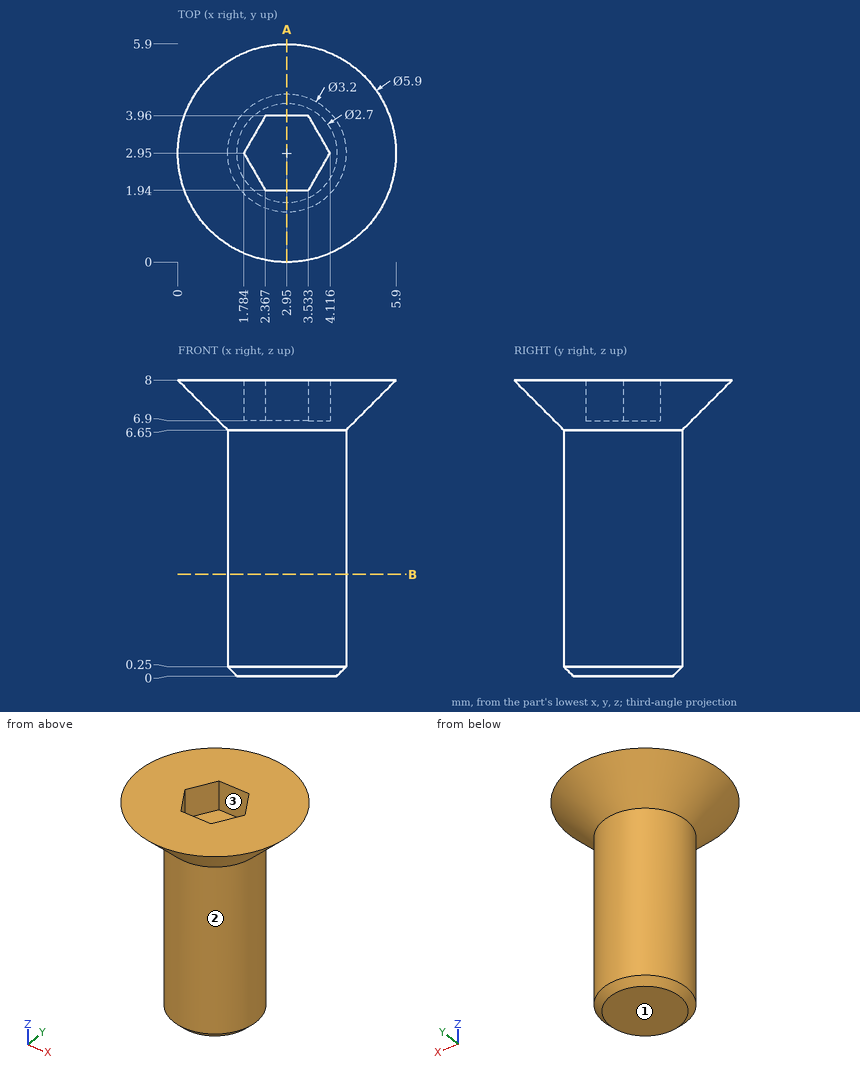
Design review of the part shown in the three views and the two pictorial views. Dimensions are in mm from the part's minimum x, y and z. A direction names the side the tool comes from. Coordinates: 2 decimals unless noted, no trailing zeros. Loops run counter-clockwise (first coordinate to the right, second up) from the corner with the lowest first, then second, coordinate; pieces in that order, holes last. Notation, with made-up numbers: (84.25, 21) - (89.25, 21) arc R25 ccw to (89.25, 46) - close; hole circle Ø6 at (65.25, 14.5). An arc over 180 degrees is marked (long way). Use a Markdown table: item, result. Add a question column.
Item 1: Tool access review of the marked faces 1, 2 and 3: name each direction out of +Z, -Z, +X, -X, +Y, -Y from which nothing blocks a thin tool from reaching the whole face with its end or side.
Item 2: For line 1 (Z direction, x = 2.95, y = 3); line 2 (Y direction, x = 3, z = 0.75); line 3 (Y direction, x = 4.2, z = 3.75), list the stretches that pass through material, from the lowest coordinate up.
Item 3: We need section B-B (z = 2.75). Give the boundary of the cut face in (x, y).
Item 4: We need section A-A (x = 2.95). Give the boundary of the cut face in (y, z).
Item 5: Insertion check: pin 1 Ø0.9 at (x, z) = (3, 7.5) entering from -Y; pin 2 Ø2 at (y, z) = (2.5, 4) entering from -X; pin 3 Ø0.5 at (x, z) = (3, 7.5) entering from +Y. Each pin has a flat end and moves straight along its axis. Give the tip position at first contact, or say it passes through.
Results list:
| question | item | result |
|---|---|---|
| 1 | face 1 | -Z, +X, -X, +Y, -Y |
| 1 | face 2 | -Z |
| 1 | face 3 | +Z |
| 2 | line 1 | z = 0 to 6.9 |
| 2 | line 2 | y = 1.35 to 4.55 |
| 2 | line 3 | y = 1.95 to 3.95 |
| 3 | outline | circle Ø3.2 at (2.95, 2.95) |
| 4 | outline | (0, 8) - (1.35, 6.65) - (1.35, 0.25) - (1.6, 0) - (4.3, 0) - (4.55, 0.25) - (4.55, 6.65) - (5.9, 8) - (3.96, 8) - (3.96, 6.9) - (1.94, 6.9) - (1.94, 8) - close |
| 5 | pin 1 | stops at y = 0.05 |
| 5 | pin 2 | stops at x = 1.35 |
| 5 | pin 3 | stops at y = 5.65 |
